Input: part model. Units: mm. Frame: model coordinates. A direction names the side the tool comes from. Give positions to 0.01 mm unless a question says otherwise; leave off trailing zeros. Order: outer loops, then holes, each group sorted by start corner. A loop starts at its lowest first (then second) coordinate and runs counter-clockwise, first axis right, second up. Notation, with made-up numbers: (27, -3) - (61, -3) arc R17 cw to (61, 15) - close; hole circle Ø9 at (3.5, 27). An arc over 180 degrees is marked (long way). Use a Markdown table: item, result.
from build123d import *

# Parameters (mm, degrees)
F2_R     = 9.525
F3_DEPTH = 6.35
F4_R     = 6.35
F5_DEPTH = 50.8
F6_SIZE  = 1.27


with BuildPart() as f3:
    # F2 (on Front) → F3 (new body)
    with BuildSketch(Plane.XZ):
        Circle(F2_R)
    extrude(amount=F3_DEPTH)

    # F4 (on Front) → F5 (join)
    with BuildSketch(Plane.XZ):
        Circle(F4_R)
    extrude(amount=-F5_DEPTH)

    # F6
    f6_edges = [f3.edges().sort_by_distance(p)[0] for p in [
        (-6.35, 50.8, 0),
    ]]
    chamfer(f6_edges, length=F6_SIZE)


solid = f3.part
1. Pin query (flat end, axial travel): pin 1 (4 mm diameter, centred on x = 1.5, y = 11, fed in from -Z); pin 2 (1 mm diameter, centred on x = -0.5, y = 26.5, fed in from +Z); pin 3 (1.5 mm diameter, centred on y = 4.5, z = -7.5, fed in from -X); pin 4 (4 mm diameter, centred on x = -2.5, z = 7, fed in from +Y). Return the tip coordinate at first contact, or that it passes through.
Response:
| item | result |
|---|---|
| pin 1 | stops at z = -6.35 |
| pin 2 | stops at z = 6.35 |
| pin 3 | passes through |
| pin 4 | stops at y = 50.45 |
2. Section query D-D (x = -7.75). Return loops of the section in (y, z).
Response:
| item | result |
|---|---|
| outline | (-6.35, -5.54) - (0, -5.54) - (0, 5.54) - (-6.35, 5.54) - close |
3. Section query C-C (y = 44). Return loops of the section in (x, z).
Response:
| item | result |
|---|---|
| outline | circle Ø12.7 at (0, 0) |
4. Material intervals for line 1 along Y through (x, z) = (7, 2); line 2 along X through (y, z) = (15.5, 1); line 3 along Z through (x, y) = (-5.25, 34.5), sorted ascending.
Response:
| item | result |
|---|---|
| line 1 | y = -6.35 to 0 |
| line 2 | x = -6.27 to 6.27 |
| line 3 | z = -3.57 to 3.57 |
5. Section query A-A (x = 0). Return loops of the section in (y, z) (3 decimals).
Response:
| item | result |
|---|---|
| outline | (-6.35, -9.525) - (0, -9.525) - (0, -6.35) - (49.53, -6.35) - (50.8, -5.08) - (50.8, 5.08) - (49.53, 6.35) - (0, 6.35) - (0, 9.525) - (-6.35, 9.525) - close |
6. Section query B-B (z = 0). Return loops of the section in (x, y) (3 decimals).
Response:
| item | result |
|---|---|
| outline | (-9.525, -6.35) - (9.525, -6.35) - (9.525, 0) - (6.35, 0) - (6.35, 49.53) - (5.08, 50.8) - (-5.08, 50.8) - (-6.35, 49.53) - (-6.35, 0) - (-9.525, 0) - close |
7. Set-up query: faces 1 (the face through (-7.559, -3.131, -5.796)), 2 (the face through (-1.38, 24.42, -6.2)). Return all of +Z, -Z, +X, -X, +Y, -Y with unobstructed straight access to the full face (end or side cutting, diameter ignored); none if empty.
Response:
| item | result |
|---|---|
| face 1 | +Y, -Y |
| face 2 | +Y |
